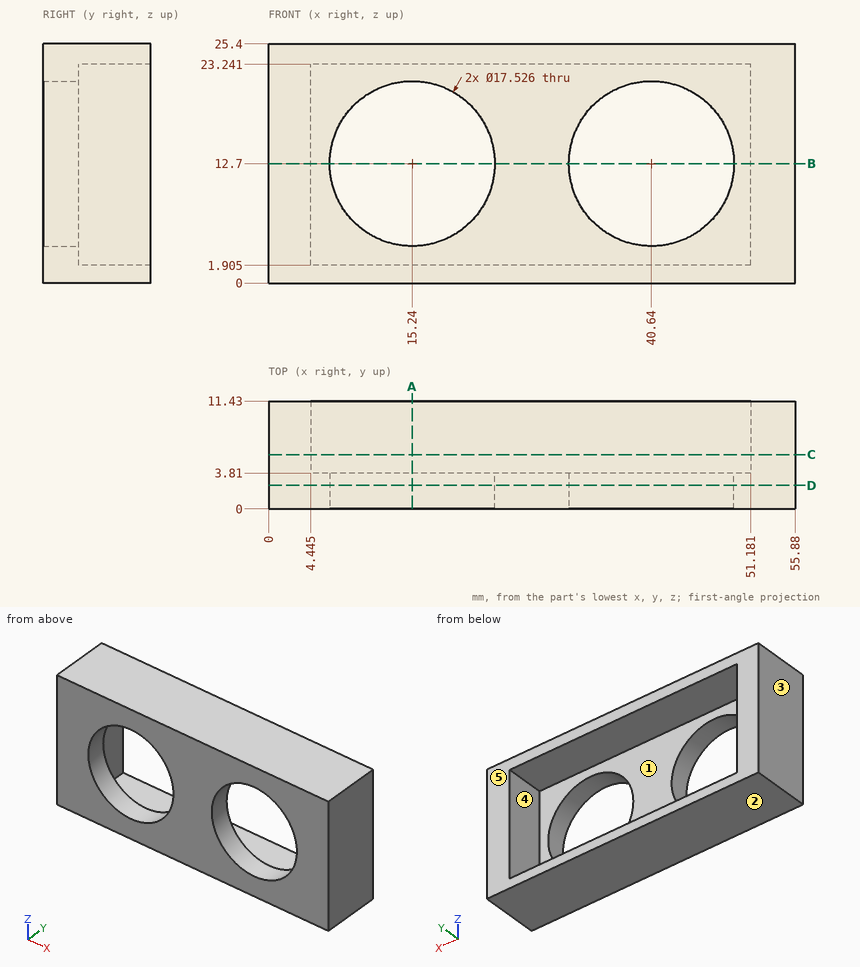
Drawing for the job (mm, zero at the part's lowest x, y, z). A direction names the side the tool comes from. Give positions to 0.01 mm unless a question says otherwise; leave off trailing zeros. Order: outer loops, then holes, each group sorted by start corner. A loop starts at its lowest first (then second) coordinate and runs counter-clockwise, first axis right, second up. Notation, with made-up numbers: (9.25, 3.25) - (53.25, 3.25) arc R17 ccw to (53.25, 12.25) - close; hole circle Ø4 at (66, 70.5). An arc over 180 degrees is marked (long way). Write item = value, one per line. Start each with the question number.
1. Cut at C-C, the plane y = 5.75. List the corners of the cut face in (x, z) (3 decimals).
2. Two-plate mould, pull along X, no slides. Class the marked faces 3, 4 and 5: pulls with the +X half, pulls with the -X half, needs draft (parallel to the pull), parting line crosses it, or undercut.
3. Drop a flat-ended pin along its axis: P1, Ø1, axis at x = 9, y = 9, coming from the -Z side. Give the stop position or say it passes through.
4. Which spindle directions (+Z, -Z, +X, -X, +Y, -Y) get a long thin tool onto all of the face, cutting with end or side? Do the marked faces 1 and 2. Say none if no direction does.
5. Cut at D-D, the plane y = 2.5. List the corners of the cut face in (x, z).
6. Cut at B-B, the plane z = 12.7. List the corners of the cut face in (x, y) (3 decimals).
7. Cut at A-A, the plane x = 15.24. List the corners of the cut face in (y, z) (3 decimals).
8. Probe line 1 along X through (y, z) = (7.75, 6.75) (3 decimals); line 2 along Z through (x, y) = (15.24, 1.45); line 3 along Z through (x, y) = (27, 9) (3 decimals). List the from-to ranges inside material, lowest first.
Taken from the geometry:
q1.outline = (0, 0) - (55.88, 0) - (55.88, 25.4) - (0, 25.4) - close; hole (4.445, 1.905) - (51.181, 1.905) - (51.181, 23.241) - (4.445, 23.241) - close
q2.face_3 = pulls with the -X half
q2.face_4 = undercut
q2.face_5 = needs draft
q3.P1 = 0
q4.face_1 = +Y
q4.face_2 = -Z, +X, -X, +Y, -Y
q5.outline = (0, 0) - (55.88, 0) - (55.88, 25.4) - (0, 25.4) - close; hole circle Ø17.53 at (15.24, 12.7); hole circle Ø17.53 at (40.64, 12.7)
q6.outline = (0, 0) - (6.477, 0) - (6.477, 3.81) - (4.445, 3.81) - (4.445, 11.43) - (0, 11.43) - close; (24.003, 0) - (31.877, 0) - (31.877, 3.81) - (24.003, 3.81) - close; (49.403, 0) - (55.88, 0) - (55.88, 11.43) - (51.181, 11.43) - (51.181, 3.81) - (49.403, 3.81) - close
q7.outline = (0, 0) - (11.43, 0) - (11.43, 1.905) - (3.81, 1.905) - (3.81, 3.937) - (0, 3.937) - close; (0, 21.463) - (3.81, 21.463) - (3.81, 23.241) - (11.43, 23.241) - (11.43, 25.4) - (0, 25.4) - close
q8.line_1 = 0 to 4.445, 51.181 to 55.88
q8.line_2 = 0 to 3.94, 21.46 to 25.4
q8.line_3 = 0 to 1.905, 23.241 to 25.4
